For this review, take the finished solid that the model builds, in its own axes (mm). Face numbers are marked on the shaded views. Give positions to 0.01 mm unless a question says otherwise; leave off trailing zeros. Loops run counter-clockwise (first coordinate to the right, second up) from the corner with the lowest first, then second, coordinate; pieces in that order, holes last.
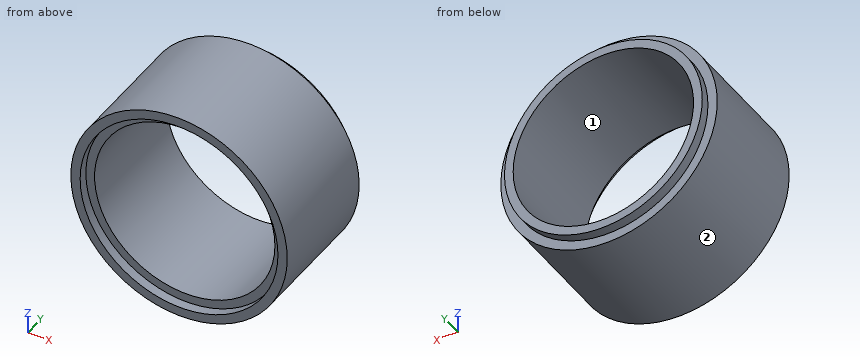
```python
from build123d import *

# Parameters (mm, degrees)
F2_R     = 46.5
F2_R_2   = 42.5
F2_R_3   = 38.75
F3_DEPTH = 54.5
F4_DEPTH = 4
F5_R     = 42.5
F5_R_2   = 38.75
F6_DEPTH = 4


with BuildPart() as f3:
    # F2 (on Front) → F3 (new body)
    with BuildSketch(Plane.XZ):
        Circle(F2_R)
        Circle(F2_R_2, mode=Mode.SUBTRACT)
        Circle(F2_R_2)
        Circle(F2_R_3, mode=Mode.SUBTRACT)
    extrude(amount=F3_DEPTH)

    # F2 (on Front) → F4 (cut)
    with BuildSketch(Plane.XZ):
        Circle(F2_R)
        Circle(F2_R_2, mode=Mode.SUBTRACT)
    extrude(amount=F4_DEPTH, mode=Mode.SUBTRACT)

    # F5 (on face) → F6 (cut)
    with BuildSketch(Plane.XZ.offset(54.5)):
        Circle(F5_R)
        Circle(F5_R_2, mode=Mode.SUBTRACT)
    extrude(amount=-F6_DEPTH, mode=Mode.SUBTRACT)


solid = f3.part
```
Item 1: For L1, parallel to Z at x = 0, y = -32.5; L2, parallel to Z at x = 0, y = -52.3; L3, parallel to X at y = -23, z = -12.5, list the stretches that pass through material, from the lowest coordinate up.
Answer:
L1: z = -46.5 to -38.75, 38.75 to 46.5
L2: z = -46.5 to -42.5, 42.5 to 46.5
L3: x = -44.79 to -36.68, 36.68 to 44.79
Item 2: Clearance check with flat-ended pins moving along their axes: pin 1 Ø6 at (y, z) = (-7.5, 17) entering from -X; pin 2 Ø2 at (x, y) = (19, -15) entering from +Z; pin 3 Ø10 at (x, y) = (12.5, -28) entering from +Z; pin 4 Ø10 at (y, z) = (-13, -3) entering from -X. State where each tip first meets the part, or that it passes through.
Answer:
pin 1: stops at x = -44.34
pin 2: stops at z = 42.87
pin 3: stops at z = 45.89
pin 4: stops at x = -46.5
Item 3: Take a section at B-B on x = 0. Give the boundary of the cut face in (y, z), and give its area (3 significant figures).
Answer:
outline: (-54.5, -46.5) - (-4, -46.5) - (-4, -42.5) - (0, -42.5) - (0, -38.75) - (-50.5, -38.75) - (-50.5, -42.5) - (-54.5, -42.5) - close; (-54.5, 42.5) - (-50.5, 42.5) - (-50.5, 38.75) - (0, 38.75) - (0, 42.5) - (-4, 42.5) - (-4, 46.5) - (-54.5, 46.5) - close
area: 783 mm2
Item 4: Take a section at A-A on z = 0. Give the boundary of the cut face in (x, y).
Answer:
outline: (-46.5, -54.5) - (-42.5, -54.5) - (-42.5, -50.5) - (-38.75, -50.5) - (-38.75, 0) - (-42.5, 0) - (-42.5, -4) - (-46.5, -4) - close; (38.75, -50.5) - (42.5, -50.5) - (42.5, -54.5) - (46.5, -54.5) - (46.5, -4) - (42.5, -4) - (42.5, 0) - (38.75, 0) - close
Item 5: The part is to be moulded in two halves that separate along X. For the marked faces 1 and 2, say which applies: released by +X, released by -X, zero draft, split by the parting line, or undercut.
Answer:
face 1: undercut
face 2: split by the parting line
Item 6: Take a section at C-C on y = -29. Give the boundary of the cut face in (x, z), and give its area (3 significant figures).
Answer:
outline: circle Ø93 at (0, 0); hole circle Ø77.5 at (0, 0)
area: 2,080 mm2
